Read the model definition and answer for the solid it produces. Units are mm, in the model's axes. A direction names the side the tool comes from. Give positions to 0.01 mm unless a question says otherwise; leave off trailing zeros. Loops run counter-clockwise (first coordinate to the right, second up) from the corner with the lowest first, then second, coordinate; pieces in that order, holes last. Notation, with made-up numbers: (-24, 39) -> (8, 39) arc R21 ccw to (8, 69) -> close; hole circle Ø3 at (47, -16.75). An arc over 180 degrees is marked (long way). Write each question's results on one line, items separated by ' | '. Start each with the question number.
Item 1: Determine the mould class of faces 5 (the flat face through (1, -13, -50)), 6 (the cylindrical face through (1.014, -37.979, 21.345)), 7 (the flat face through (1, 0, -33)), 8 (the flat face through (1, -25, 44)) for opening direction Y: +Y half, -Y half, draft (parallel to the pull), parting line (faces both ways), or undercut.
Item 2: Each of these flat-tipped pins is pushed along its axis until it touches: P1, Ø2, axis at y = -20, z = -2.5, coming from the -X side; P2, Ø0.6, axis at x = 0.5, z = -24.5, coming from the -Y side; P3, Ø1, axis at x = 0.5, z = -8.5, coming from the +Y side. Where does it stop, or does it pass through?
Item 3: Section B-B on x = 1.55 is taken. State how many separate pieces and enclosed holes the cut face has, and give its area (3 significant figures).
Item 4: Find the intervals of material crossed by line 1 (Y direction, x = 0.8, z = -2.5); line 2 (Z direction, x = 0.15, y = -21); line 3 (Y direction, x = 0.8, z = 42.5), in increasing order.
Item 5: Which of the six approach directions +Z, -Z, +X, -X, +Y, -Y give full straight-line access (tool end or side, diameter ignored) to faces 1 (the flat face through (1, -35, -2)), 2 (the flat face through (2, -19.8, 11.8)), 3 (the flat face through (1.01, -12.67, -21.06)), 4 (the cylindrical face through (0.986, -35.782, 29.975))?
Item 6: Section A-A on z = 16.5 is taken. Write down the section's boundary in (x, y), and give its area (3 significant figures).
Autodesk Inventor part; units mm, degrees
ref_plane "YZ Plane" through (0, 0, 0) normal (1, 0, 0) x (0, 1, 0)
ref_plane "XZ Plane" through (0, 0, 0) normal (0, 1, 0) x (-1, 0, 0)
ref_plane "XY Plane" through (0, 0, 0) normal (0, 0, 1) x (1, 0, 0)
sketch "スケッチ1" plane through (0, 0, 0) normal (1, 0, 0) x (0, 1, 0)
  line L0 (0, 50) -> (-50, 50)
  line L1 (-50, 50) -> (-50, -50)
  line L2 (-50, -50) -> (0, -50)
  line L3 (0, -50) -> (0, 50)
  point P0 (0, 0)
  dimension "d0" = 50
  dimension "d2" = 100
  dimension "d3" = 50
  dimension "d4" = 50
extrude "押し出し1" add sketch "スケッチ1" along normal blind 2
sketch "スケッチ2" plane through (2, 0, 0) normal (1, 0, 0) x (0, 0, -1)
  line L0 (-50, 0) -> (-50, -50)
  line L1 (-50, -50) -> (50, -50)
  line L2 (50, -50) -> (50, 0)
  line L3 (50, 0) -> (-50, 0)
  line L4 (-25, -50) -> (-10, -35)
  line L5 (-10, -35) -> (15, -35)
  line L6 (15, -35) -> (50, -25.6218)
  line L7 (-50, 0) -> (-25, 0)
  line L8 (-25, 0) -> (-10, -15)
  line L9 (-10, -15) -> (12.367, -15)
  line L10 (12.367, -15) -> (30, -10.2752)
  line L11 (30, -10.2752) -> (30, 0)
  line L12 (-25, -50) -> (-50, -50)
  line L13 (-50, -50) -> (-50, 0)
  point P0 (0, 0)
  dimension "d7" = 135
  dimension "d8" = 135
  dimension "d9" = 25
  dimension "d10" = 25
  dimension "d11" = 50
  dimension "d16" = 165
  dimension "d17" = 20
  dimension "d18" = 20
  dimension "d89" = 20
  dimension "d90" = 25
extrude "押し出し2" cut sketch "スケッチ2" against normal blind 2 contours L3 L8 L9 L10 L11 L2 L6 L5 L4 L1 L0 keep common part
sketch "スケッチ3" plane through (2, 0, 0) normal (1, 0, 0) x (0, 0, -1)
  line L0 (30, -10.2752) -> (30, 0)
  line L1 (12.367, -15) -> (30, -10.2752)
  line L2 (-10, -15) -> (12.367, -15)
  line L3 (-25, 0) -> (-10, -15)
  line L4 (-25, 0) -> (-50, 0)
  line L5 (-50, 0) -> (-50, -50)
  line L6 (-50, -50) -> (-25, -50)
  line L7 (-10, -35) -> (-25, -50)
  line L8 (15, -35) -> (-10, -35)
  line L9 (50, -25.6218) -> (15, -35)
  line L10 (50, -25.6218) -> (50, 0)
  line L11 (50, 0) -> (30, 0)
  circle A0 centre (-42.5, -7.5) radius 2
  circle A1 centre (-42.5, -42.5) radius 2
  circle A2 centre (-22.5, -12.5) radius 1.25
  circle A3 centre (-22.5, -37.5) radius 1.25
  arc A4 (36, -4) -> (44, -4) centre (40, -4) ccw
  line L12 (36, -4) -> (36, 0)
  line L13 (44, -4) -> (44, 0)
  point P0 (0, 0)
  dimension "d21" = 8
  dimension "d25" = 4
  dimension "d30" = 6
  dimension "d31" = 4
  dimension "d35" = 25
  dimension "d36" = 35
  dimension "d37" = 12.5
  dimension "d38" = 7.5
  dimension "d40" = 7.5
  dimension "d41" = 7.5
  dimension "d61" = 2.5
  dimension "d68" = 20
  dimension "d69" = 20
extrude "押し出し5" cut sketch "スケッチ3" against normal blind 2 contours L0 L11 L12 A4 L13 L10 L9 L8 L7 L6 L5 L4 L3 L2 L1 keep common part
sketch "スケッチ4" plane through (2, 0, 0) normal (1, 0, 0) x (0, 0, -1)
  line L0 (50, 0) -> (30, 0)
  circle A0 centre (33, -4) radius 1
  arc A1 (36, -4) -> (44, -4) centre (40, -4) ccw
  point P0 (0, 0)
  dimension "d47" = 4
  dimension "d49" = 2
  dimension "d64" = 7
hole "穴1" at (2, -4, -33) direction (-1, 0, 0) diameter 2 end through all
pattern_circular "円形状パターン2" count 5 over 180 about axis through (2, -4, -40) along (1, 0, 0) of "穴1"
sketch "スケッチ5" plane through (2, 0, 0) normal (1, 0, 0) x (0, 0, -1)
  line L0 (-10, -15) -> (12.367, -15)
  circle A0 centre (-22.5, -12.5) radius 1.25
  circle A1 centre (-22.5, -37.5) radius 1.25
  circle A2 centre (2.5, -20) radius 1.3
  circle A3 centre (2.5, -30) radius 1.3
  point P0 (0, 0)
  dimension "d70" = 2.6
  dimension "d74" = 5
  dimension "d75" = 10
  dimension "d91" = 25
  dimension "d92" = 25
hole "穴2" at (2, -20, -2.5) at (2, -30, -2.5) direction (-1, 0, 0) diameter 2.2 end through all
sketch "スケッチ7" plane through (2, 0, 0) normal (1, 0, 0) x (0, 0, -1)
  line L0 (-10, -15) -> (12.367, -15)
  line L1 (-25, 0) -> (-50, 0)
  line L2 (-50, 0) -> (-50, -50)
  line L3 (15, -35) -> (-10, -35)
  line L4 (-18.0096, -30) -> (-8.0096, -30)
  line L5 (-8.0096, -30) -> (-8.0089, -20)
  line L6 (-18.0089, -20) -> (-31, -12.5)
  line L7 (-31, -12.5) -> (-31, -37.5)
  line L8 (-31, -37.5) -> (-18.0096, -30)
  line L9 (-18.0089, -20) -> (-8.0089, -20)
  point P0 (0, 0)
  dimension "d94" = 10
  dimension "d99" = 150
  dimension "d102" = 5
  dimension "d103" = 5
  dimension "d104" = 25
  dimension "d105" = 12.5
  dimension "d106" = 19
extrude "押し出し7" cut sketch "スケッチ7" against normal blind 2
sketch "スケッチ8" plane through (2, 0, 0) normal (1, 0, 0) x (0, 0, -1)
  line L0 (-25, 0) -> (-50, 0)
  line L1 (-50, 0) -> (-50, -50)
  line L2 (50, 0) -> (44, 0)
  line L3 (-44, -15) -> (-44, -35)
  line L4 (-44, -15) -> (-36, -10.3812)
  line L5 (-36, -10.3812) -> (-36, -39.6188)
  line L6 (-44, -35) -> (-36, -39.6188)
  point P0 (0, 0)
  dimension "d111" = 120
  dimension "d112" = 120
  dimension "d113" = 20
  dimension "d115" = 8
  dimension "d116" = 14
  dimension "d117" = 15
extrude "押し出し8" cut sketch "スケッチ8" against normal blind 2
fillet "フィレット1" radius 10 2 edges at (1, -20, 18.0089) (1, -30, 18.0096)
fillet "フィレット2" radius 2 8 edges at (1, -30, 8.0096) (1, -12.5, 31) (1, -20, 8.0089) (1, -10.3812, 36) (1, -35, 44) (1, -15, 44) (1, -37.5, 31) (1, -39.6188, 36)
sketch "スケッチ10" plane through (2, 0, 0) normal (1, 0, 0) x (0, 0, -1)
  line L0 (-10, -15) -> (12.367, -15)
  line L1 (15, -35) -> (-10, -35)
  line L2 (50, 0) -> (44, 0)
  line L3 (12, -20) -> (42, -20)
  line L4 (42, -20) -> (14.5252, -30)
  line L5 (14.5252, -30) -> (12, -20)
  point P0 (0, 0)
  dimension "d124" = 30
  dimension "d127" = 160
  dimension "d128" = 5
  dimension "d129" = 5
  dimension "d130" = 12
extrude "押し出し9" cut sketch "スケッチ10" against normal blind 2
fillet "フィレット3" radius 2 3 edges at (1, -20, -12) (1, -20, -42) (1, -30, -14.5252)
properties part number "Arm_MiniLink_1" material "アルミニウム 6061"
Findings:
1) face 5: draft | face 6: undercut | face 7: +Y half | face 8: undercut
2) P1: through | P2: y = -32.53 | P3: y = -15
3) separate pieces: 1 | enclosed holes: 14 | area: 2,390 mm2
4) line 1: -35 to -31.1, -28.9 to -21.1, -18.9 to -15 | line 2: -50 to -32.39, -12.84 to -2.96, -2.04 to 8.28, 31 to 36, 44 to 50 | line 3: -50 to -44.5, -40.5 to -35.87, -14.13 to -9.5, -5.5 to 0
5) face 1: -Z, +X, -X, -Y | face 2: +Z, -Z, +X, +Y, -Y | face 3: +X, -X, +Y | face 4: +X, -X
6) outline: (0, -41.5) -> (2, -41.5) -> (2, -30.07) -> (0, -30.07) -> close; (0, -19.93) -> (2, -19.93) -> (2, -8.5) -> (0, -8.5) -> close | area: 45.7 mm2
